Part print with two shaded views. Sizes in mm from the minimum x, y, z corner. Round coordinates to 2 decimals unless told otherwise and drop trailing zeros. Order: outer loops, then holes, each group sorted by start corner. A loop starts at its lowest first (then second) coordinate and runs counter-clockwise, first axis right, second up. Notation, with made-up numbers: (47.5, 33) -> (82.5, 33) arc R21 ccw to (82.5, 59) -> close; hole circle Ø4 at (37, -0.75). An arc over 180 degrees is marked (long way). Put each result on its own line as item: value. Start each with the question number.
Q1. Cut at C-C, the plane x = 62. List the corners of the cut face in (y, z).
Q2. Cut at A-A, the plane y = 0.6. State how many separate pieces and enclosed holes the cut face has, and give its area (3 significant figures).
Q3. Flat gauge pins, fed straight in: P1, Ø1.5, axis at x = 4.5, y = 2, coming from the +Z side; P2, Ø1.5, axis at x = 94, y = 1, coming from the -Z side; P3, Ø1.5, axis at y = 1.5, z = 56.5, coming from the +X side. Where does each tip first touch, or does it go through?
Q4. Cut at B-B, the plane z = 40.5. List the corners of the cut face in (x, y).
Q5. Probe L1, parallel to Z at x = 90.5, y = 1.1; L2, parallel to X at y = 1.3, z = 19.25; L3, parallel to X at y = 1.9, z = 21.5. List the from-to ranges inside material, lowest first.
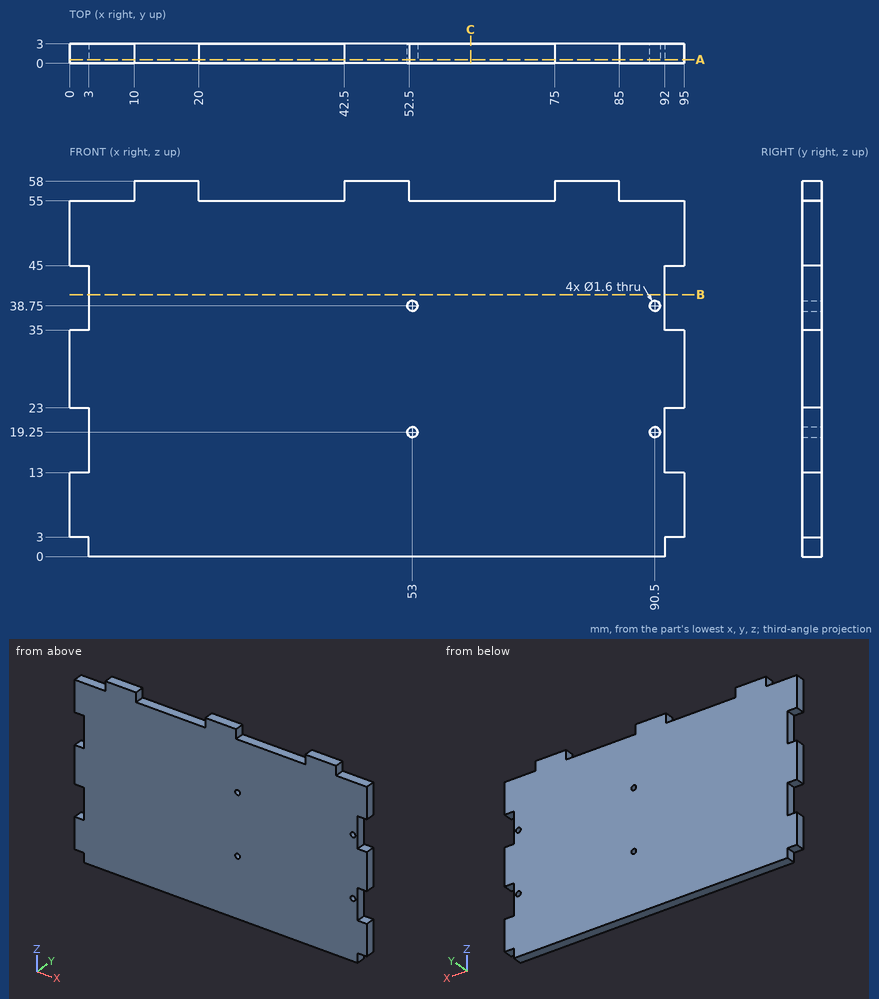
Ans:
1. outline: (0, 0) -> (3, 0) -> (3, 55) -> (0, 55) -> close
2. separate pieces: 1
2. enclosed holes: 4
2. area: 5,170 mm^2
3. P1: stops at z = 55
3. P2: stops at z = 3
3. P3: stops at x = 85
4. outline: (3, 0) -> (92, 0) -> (92, 3) -> (3, 3) -> close
5. L1: z = 0 to 18.45, 20.05 to 37.95, 39.55 to 55
5. L2: x = 3 to 52.2, 53.8 to 89.7, 91.3 to 92
5. L3: x = 3 to 92
